Source: CAD feature listing. Evaluate the final solid. Frame: model axes, mm. A direction names the side the tool comes from. Round coordinates to 2 decimals unless told otherwise and drop trailing zeros. Loops run counter-clockwise (first coordinate to the right, second up) from the corner with the lowest first, then second, coordinate; pieces in that order, holes last.
(1) Section B-B, the plane x = -12.5. Return the cut outline in (y, z).
(2) Section A-A, the plane y = -6.45. Return the cut outline in (x, z), plus the area to 3 significant figures.
(3) Section C-C, the plane x = 15. Return the cut outline in (y, z), plus the area to 3 significant figures.
(4) First-contact query: pin 1 Ø6.5 at (x, z) = (-12.5, 15) entering from -Y. Flat tip, straight axial feed; report the tip coordinate or a pass-through.
(5) Set-up query: faces 4 (the flat face through (-21.5, -6.7, -14)), 5 (the cylindrical face through (20.733, -7.028, -8.841)). Return all of +Z, -Z, +X, -X, +Y, -Y with unobstructed straight access to the full face (end or side cutting, diameter ignored); none if empty.
(6) Material intervals for probe 1 along Z at (x, y) = (-12.5, -4.4); probe 2 along X at (y, z) = (-6.15, -8); probe 3 along X at (y, z) = (-8.2, -5.5), sorted ascending.
(7) Mould query, pull axis Z, two halves, no side actions, for faces 1 (the flat face through (-21.5, -6.7, 19)), 2 (the cylindrical face through (12.24, -4.014, 16.983)), 3 (the flat face through (21.5, -3.7, -14)). Classes: pulls with the +Z half, pulls with the -Z half, needs draft (parallel to the pull), parting line crosses it, or undercut.
```python
from build123d import *

# Parameters (mm, degrees)
F0_W      = 45
F0_H      = 35
F1_DEPTH  = 4.5
F2_W      = 15
F2_H      = 1.5
F3_DEPTH  = 35.001
F4_R      = 1.75
F5_DEPTH  = 3.5
F6_R      = 2
F7_DEPTH  = 4.501
F8_W      = 10
F8_H      = 10
F9_DEPTH  = 3
F10_SIZE  = 2
F11_W     = 48.3506806195
F11_H     = 3
F12_DEPTH = 35.001
F13_W     = 45
F13_H     = 35
F14_DEPTH = 4.5
F15_SIZE  = 1.99999
F16_R     = 2
F17_DEPTH = 6.001
F18_R     = 3.5
F19_DEPTH = 4
F20_R     = 3.5
F21_DEPTH = 4
F22_R     = 2
F23_DEPTH = 6.001


# Not quite as in the source:
# - a fillet or chamfer is up to 0.001 mm smaller than in the source, because OpenCascade refuses the exact size


with BuildPart() as f1:
    # F0 (on Front) → F1 (new body)
    with BuildSketch(Plane.XZ):
        with Locations((0, 2.5)):
            Rectangle(F0_W, F0_H)
    extrude(amount=F1_DEPTH)

    # F2 (on face) → F3 (cut, through all)
    with BuildSketch(Plane.XY.offset(20)):
        with Locations((-2.5, -2.25)):
            Rectangle(F2_W, F2_H)
    extrude(amount=-F3_DEPTH, mode=Mode.SUBTRACT)

    # F4 (on face) → F5 (cut)
    with BuildSketch(Plane.XZ.offset(4.5)):
        with Locations((17.5, -7.5)):
            Circle(F4_R)
        with Locations((-17.5, -7.5)):
            Circle(F4_R)
    extrude(amount=-F5_DEPTH, mode=Mode.SUBTRACT)

    # F6 (on face) → F7 (cut, through all)
    with BuildSketch(Plane.XZ.offset(4.5)):
        with Locations((17.5, -7.5)):
            Circle(F6_R)
        with Locations((-17.5, -7.5)):
            Circle(F6_R)
    extrude(amount=-F7_DEPTH, mode=Mode.SUBTRACT)

    # F8 (on face) → F9 (cut)
    with BuildSketch(Plane(origin=(0, 0, 0), x_dir=(-1, 0, 0), z_dir=(0, 1, 0))):
        with Locations((5, 10)):
            Rectangle(F8_W, F8_H)
    extrude(amount=-F9_DEPTH, mode=Mode.SUBTRACT)

    # F10
    f10_edges = [f1.edges().sort_by_distance(p)[0] for p in [
        (-22.5, -2.25, 20),
        (22.5, -2.25, 20),
        (22.5, -2.25, -15),
        (-22.5, -2.25, -15),
    ]]
    chamfer(f10_edges, length=F10_SIZE)

    # F11 (on face) → F12 (cut, through all)
    with BuildSketch(Plane(origin=(0, 0, -15), x_dir=(1, 0, 0), z_dir=(0, 0, -1))):
        with Locations((0.253405422, 1.5)):
            Rectangle(F11_W, F11_H)
    extrude(amount=-F12_DEPTH, mode=Mode.SUBTRACT)

    # F13 (on face) → F14 (join)
    with BuildSketch(Plane.XZ.offset(4.5)):
        with Locations((0, 2.5)):
            Rectangle(F13_W, F13_H)
    extrude(amount=F14_DEPTH)

    # F15 (size 2 in the source; OpenCascade refuses exactly that, so slightly less here)
    f15_edges = [f1.edges().sort_by_distance(p)[0] for p in [
        (-22.5, -6.75, -15),
        (22.5, -6.75, -15),
        (22.5, -6.75, 20),
        (-22.5, -6.75, 20),
    ]]
    chamfer(f15_edges, length=F15_SIZE)

    # F16 (on face) → F17 (cut, through all)
    with BuildSketch(Plane(origin=(0, -3, 0), x_dir=(-1, 0, 0), z_dir=(0, 1, 0))):
        with Locations((17.5, -7.5)):
            Circle(F16_R)
        with Locations((-17.5, -7.5)):
            Circle(F16_R)
    extrude(amount=-F17_DEPTH, mode=Mode.SUBTRACT)

    # F18 (on face) → F19 (cut)
    with BuildSketch(Plane.XZ.offset(9)):
        with Locations((-17.5, -7.5)):
            Circle(F18_R)
        with Locations((17.5, -7.5)):
            Circle(F18_R)
    extrude(amount=-F19_DEPTH, mode=Mode.SUBTRACT)

    # F20 (on face) → F21 (cut)
    with BuildSketch(Plane.XZ.offset(9)):
        with Locations((-12.5, 15)):
            Circle(F20_R)
        with Locations((12.5, 15)):
            Circle(F20_R)
    extrude(amount=-F21_DEPTH, mode=Mode.SUBTRACT)

    # F22 (on face) → F23 (cut, through all)
    with BuildSketch(Plane.XZ.offset(9)):
        with Locations((-12.5, 15)):
            Circle(F22_R)
        with Locations((12.5, 15)):
            Circle(F22_R)
    extrude(amount=-F23_DEPTH, mode=Mode.SUBTRACT)


solid = f1.part
```
Output values:
1. outline: (-9, -15) - (-3, -15) - (-3, 13) - (-5, 13) - (-5, 11.5) - (-9, 11.5) - close; (-9, 18.5) - (-5, 18.5) - (-5, 17) - (-3, 17) - (-3, 20) - (-9, 20) - close
2. outline: (-22.5, -13) - (-20.5, -15) - (20.5, -15) - (22.5, -13) - (22.5, 18) - (20.5, 20) - (-20.5, 20) - (-22.5, 18) - close; hole circle Ø7 at (-17.5, -7.5); hole circle Ø7 at (-12.5, 15); hole circle Ø7 at (12.5, 15); hole circle Ø7 at (17.5, -7.5)
2. area: 1,410 mm2
3. outline: (-9, -15) - (-3, -15) - (-3, 20) - (-9, 20) - (-9, 17.45) - (-5, 17.45) - (-5, 12.55) - (-9, 12.55) - (-9, -5.05) - (-5, -5.05) - (-5, -9.95) - (-9, -9.95) - close
3. area: 171 mm2
4. pin 1: stops at y = -5
5. face 4: -Z, -X, +Y, -Y
5. face 5: -Y
6. probe 1: z = -15 to 13, 17 to 20
6. probe 2: x = -22.5 to -20.96, -14.04 to 14.04, 20.96 to 22.5
6. probe 3: x = -22.5 to -20.37, -14.63 to 14.63, 20.37 to 22.5
7. face 1: pulls with the +Z half
7. face 2: undercut
7. face 3: pulls with the -Z half
